Input: part model. Units: mm. Frame: model coordinates. A direction names the side the tool comes from. Round coordinates to 2 decimals unless told otherwise and drop trailing zeros. Loops run counter-clockwise (first coordinate to the right, second up) from the corner with the lowest first, then second, coordinate; pieces in that order, holes last. Notation, with made-up numbers: (37, 32) -> (65, 32) arc R17 cw to (65, 41) -> close; hole circle Ø9 at (3, -29.75). An arc over 180 degrees is marked (long way). Answer as a JSON object with one key per item and string values. Group by question number.
Item 1: Set-up query: faces 5 (the flat face through (51, -7, 6)), 6 (the flat face through (-14.528, -68.878, 1.972)), 7 (the cylindrical face through (46.244, -6.856, 4.986)). Return all of +Z, -Z, +X, -X, +Y, -Y with unobstructed straight access to the full face (end or side cutting, diameter ignored); none if empty.
Item 2: Section query C-C on x = 0. Return loops of the section in (y, z).
Item 3: Section query A-A on y = -48. Return loops of the section in (x, z), and give its area (3 significant figures).
Item 4: Material intervals for line 1 (Y direction, x = -45, z = 5.1); line 2 (X direction, y = -11, z = 3.8); line 3 (X direction, y = -38, z = 1.7), sorted ascending. Write a range as [from, to].
Item 5: Section query B-B on z = 2.3. Return loops of the section in (x, y) (3 decimals).
Item 6: Pin query (flat end, axial travel): pin 1 (1.6 mm diameter, centred on x = -49.5, z = 5, fed in from +Y); pin 2 (0.6 mm diameter, centred on y = -12, z = 4.5, fed in from -X); pin 3 (0.6 mm diameter, centred on x = -42.5, z = 5.5, fed in from -Y). Return the tip coordinate at first contact, or that it passes through.
Item 7: Section query D-D on x = 16.5. Return loops of the section in (y, z), and give its area (3 significant figures).
Item 8: Draft query along X for faces 1 (the cylindrical face through (24.9, -13.1, 5)), 2 (the cylindrical face through (0.39, 48.59, 1.97)), 3 (the cylindrical face through (71.39, 14.27, 1.97)), 4 (the flat face through (62, 4, 6)). Return one class per face: released by +X, released by -X, zero draft, split by the parting line, or undercut.
from build123d import *

# Parameters (mm, degrees)
PAD_DEPTH     = 4
FILLET_R      = 5
SKETCH001_R   = 7.25
SKETCH001_R_2 = 5.75
SKETCH001_R_3 = 4.5
PAD001_DEPTH  = 2


with BuildPart() as part:
    # Sketch → Pad (new body)
    with BuildSketch(Plane.XY):
        with BuildLine():
            Line((-8.392638, -94.773898), (-20.838068, -42.247688))
            ThreePointArc((-20.838068, -42.247688), (-25.283831, -34.851678), (-33.189712, -31.392947))
            Line((-48.108948, -29.838473), (-33.189712, -31.392947))
            ThreePointArc((-48.108948, -29.838473), (-50.544507, -30.499468), (-51.902377, -32.626684))
            Line((-51.902377, -32.626684), (-59.045734, -67.993001))
            ThreePointArc((-75.934928, -68.086092), (-67.452461, -74.910237), (-59.045734, -67.993001))
            ThreePointArc((-74.580399, -5), (-78.929877, -36.4642), (-75.934928, -68.086092))
            ThreePointArc((-56.5, 27.708302), (-71.255629, 14.513509), (-74.580399, -5))
            Line((-56.5, 27.708302), (-38.027799, 35.374969))
            ThreePointArc((-38.027799, 35.374969), (-35.024382, 37.16978), (-32.660861, 39.74963))
            Line((-32.660861, 39.74963), (-29.375, 44.589632))
            ThreePointArc((29.375, 44.589632), (0, 48.589632), (-29.375, 44.589632))
            Line((32.660861, 39.74963), (29.375, 44.589632))
            ThreePointArc((32.660861, 39.74963), (35.024382, 37.16978), (38.027799, 35.374969))
            Line((56.5, 27.708302), (38.027799, 35.374969))
            ThreePointArc((74.580399, -5), (71.255629, 14.513509), (56.5, 27.708302))
            ThreePointArc((75.934928, -68.086092), (78.929877, -36.4642), (74.580399, -5))
            ThreePointArc((59.045729, -67.992978), (67.452449, -74.910237), (75.934928, -68.086092))
            Line((51.902377, -32.626684), (59.045729, -67.992978))
            ThreePointArc((51.902377, -32.626684), (50.544507, -30.499468), (48.108948, -29.838472))
            Line((33.189712, -31.392947), (48.108948, -29.838472))
            ThreePointArc((33.189712, -31.392947), (25.283831, -34.851678), (20.838068, -42.247688))
            Line((8.392638, -94.773899), (20.838068, -42.247688))
            ThreePointArc((-8.392638, -94.773898), (0, -101.410368), (8.392638, -94.773899))
        make_face()
    extrude(amount=PAD_DEPTH)

    # Fillet
    fillet_edges = [part.edges().sort_by_distance(p)[0] for p in [
        (29.375, 44.589632, 2),
        (-29.375, 44.589632, 2),
    ]]
    fillet(fillet_edges, radius=FILLET_R)

    # Sketch001 (on Face26 of Pad) → Pad001 (join)
    with BuildSketch(Plane.XY.offset(4)):
        with Locations((0, -37.310368)):
            Circle(SKETCH001_R)
        with Locations((37.833116, -19.159138)):
            Circle(SKETCH001_R_2)
        with Locations((26.165854, -7.491876)):
            Circle(SKETCH001_R_2)
        with Locations((50.739369, 14.945877)):
            Circle(SKETCH001_R_3)
        with Locations((61.739369, 3.945877)):
            Circle(SKETCH001_R_3)
        with Locations((50.739369, -7.054123)):
            Circle(SKETCH001_R_3)
        with Locations((39.739369, 3.945877)):
            Circle(SKETCH001_R_3)
        with BuildLine():
            Line((-45.578289, -0.5285), (-45.578289, 7.4715))
            ThreePointArc((-45.578289, 7.4715), (-45.871183, 8.178607), (-46.578289, 8.4715))
            Line((-46.578289, 8.4715), (-51.578289, 8.4715))
            ThreePointArc((-51.578289, 8.4715), (-52.285396, 8.178607), (-52.578289, 7.4715))
            Line((-52.578289, 7.4715), (-52.578289, -0.5285))
            Line((-52.578289, -0.5285), (-60.578289, -0.5285))
            ThreePointArc((-60.578289, -0.5285), (-61.285396, -0.821393), (-61.578289, -1.5285))
            Line((-61.578289, -1.5285), (-61.578289, -6.5285))
            ThreePointArc((-61.578289, -6.5285), (-61.285396, -7.235607), (-60.578289, -7.5285))
            Line((-60.578289, -7.5285), (-52.578289, -7.5285))
            Line((-52.578289, -7.5285), (-52.578289, -15.5285))
            ThreePointArc((-52.578289, -15.5285), (-52.285396, -16.235607), (-51.578289, -16.5285))
            Line((-51.578289, -16.5285), (-46.578289, -16.5285))
            ThreePointArc((-46.578289, -16.5285), (-45.871183, -16.235607), (-45.578289, -15.5285))
            Line((-45.578289, -15.5285), (-45.578289, -7.5285))
            Line((-45.578289, -7.5285), (-37.578289, -7.5285))
            ThreePointArc((-37.578289, -7.5285), (-36.871183, -7.235607), (-36.578289, -6.5285))
            Line((-36.578289, -6.5285), (-36.578289, -1.5285))
            ThreePointArc((-36.578289, -1.5285), (-36.871183, -0.821393), (-37.578289, -0.5285))
            Line((-37.578289, -0.5285), (-45.578289, -0.5285))
        make_face()
    extrude(amount=PAD001_DEPTH)


solid = part.part
Solved:
{
 "1": {"face 5": "+Z, +X, -X, +Y, -Y", "face 6": "+Z, -Z, -Y", "face 7": "+Z"},
 "2": {"outline": "(-101.41, 0) -> (48.59, 0) -> (48.59, 4) -> (-30.06, 4) -> (-30.06, 6) -> (-44.56, 6) -> (-44.56, 4) -> (-101.41, 4) -> close"},
 "3": {"outline": "(-78.69, 0) -> (-55.01, 0) -> (-55.01, 4) -> (-78.69, 4) -> close; (-19.48, 0) -> (19.48, 0) -> (19.48, 4) -> (-19.48, 4) -> close; (55.01, 0) -> (78.69, 0) -> (78.69, 4) -> (55.01, 4) -> close", "area": "345 mm²"},
 "4": {"line 1": "[-7.53, -0.53]", "line 2": "[-75.99, 75.99]", "line 3": "[-78.95, -52.99], [-22.61, 22.61], [52.99, 78.95]"},
 "5": {"outline": "(-75.935, -68.086) arc R8.625 ccw to (-59.046, -67.993) -> (-51.902, -32.627) arc R3.5 cw to (-48.109, -29.838) -> (-33.19, -31.393) arc R14.207 cw to (-20.838, -42.248) -> (-8.393, -94.774) arc R8.625 ccw to (8.393, -94.774) -> (20.838, -42.248) arc R14.207 cw to (33.19, -31.393) -> (48.109, -29.838) arc R3.5 cw to (51.902, -32.627) -> (59.046, -67.993) arc R8.625 ccw to (75.935, -68.086) arc R137.34 ccw to (74.58, -5) arc R30 ccw to (56.5, 27.708) -> (38.028, 35.375) arc R12.087 cw to (32.661, 39.75) -> (30.42, 43.051) arc R5 ccw to (27.536, 45.083) arc R109.861 ccw to (-27.536, 45.083) arc R5 ccw to (-30.42, 43.051) -> (-32.661, 39.75) arc R12.087 cw to (-38.028, 35.375) -> (-56.5, 27.708) arc R30 ccw to (-74.58, -5) arc R137.34 ccw to start"},
 "6": {"pin 1": "y = 8.47", "pin 2": "x = -52.58", "pin 3": "y = -7.53"},
 "7": {"outline": "(-60.56, 0) -> (47.34, 0) -> (47.34, 4) -> (-60.56, 4) -> close", "area": "432 mm²"},
 "8": {"face 1": "undercut", "face 2": "split by the parting line", "face 3": "released by +X", "face 4": "zero draft"}
}
